Geometry: final body of the model. Coordinates: model frame, mm. Give positions to 0.01 mm unless a question says otherwise; leave off trailing zeros. Order: outer loops, then holes, each group sorted by start corner. A loop starts at its lowest first (then second) coordinate and runs counter-clockwise, first axis right, second up. Notation, with made-up numbers: M 69.25,-34 L 104.25,-34 A18 ccw 104.25,-12 Z; hole C 36.25,5 d10. An arc over 180 degrees is marked long. Use CSV: the item, a comma, the result in double quotes.
```python
from build123d import *

# Parameters (mm, degrees)
SKETCH1_W           = 50.8
SKETCH1_H           = 127
BOSS_EXTRUDE1_DEPTH = 6.35
SKETCH2_R           = 5.08
CUT_EXTRUDE1_DEPTH  = 137.930502446
SKETCH3_W           = 19.05
SKETCH3_H           = 6.35
SKETCH3_R           = 1.524
BOSS_EXTRUDE2_DEPTH = 6.35
BOSS_EXTRUDE3_DEPTH = 6.35
SKETCH5_R           = 1.524
CUT_EXTRUDE2_DEPTH  = 146.219377151


with BuildPart() as part:
    # Sketch1 → Boss-Extrude1 (new body)
    with BuildSketch(Plane.XY):
        with Locations((25.4, 63.5)):
            Rectangle(SKETCH1_W, SKETCH1_H)
    extrude(amount=BOSS_EXTRUDE1_DEPTH)

    # Sketch2 → Cut-Extrude1 (cut, through all)
    with BuildSketch(Plane.XY.offset(6.35)):
        with Locations(Location((6.35, 98.072222222, 0), (0, 0, 180))):
            Circle(SKETCH2_R)
        with Locations(Location((19.05, 98.072222222, 0), (0, 0, 180))):
            Circle(SKETCH2_R)
        with Locations(Location((31.75, 98.072222222, 0), (0, 0, 180))):
            Circle(SKETCH2_R)
        with Locations(Location((44.45, 98.072222222, 0), (0, 0, 180))):
            Circle(SKETCH2_R)
        with Locations(Location((12.7, 86.783333333, 0), (0, 0, 180))):
            Circle(SKETCH2_R)
        with Locations(Location((25.4, 86.783333333, 0), (0, 0, 180))):
            Circle(SKETCH2_R)
        with Locations(Location((38.1, 86.783333333, 0), (0, 0, 180))):
            Circle(SKETCH2_R)
        with Locations(Location((44.45, 75.494444444, 0), (0, 0, 180))):
            Circle(SKETCH2_R)
        with Locations(Location((31.75, 75.494444444, 0), (0, 0, 180))):
            Circle(SKETCH2_R)
        with Locations(Location((19.05, 75.494444444, 0), (0, 0, 180))):
            Circle(SKETCH2_R)
        with Locations(Location((6.35, 75.494444444, 0), (0, 0, 180))):
            Circle(SKETCH2_R)
        with Locations(Location((6.35, 30.338888889, 0), (0, 0, 180))):
            Circle(SKETCH2_R)
        with Locations(Location((19.05, 30.338888889, 0), (0, 0, 180))):
            Circle(SKETCH2_R)
        with Locations(Location((31.75, 30.338888889, 0), (0, 0, 180))):
            Circle(SKETCH2_R)
        with Locations((19.05, 120.65)):
            Circle(SKETCH2_R)
        with Locations((6.35, 120.65)):
            Circle(SKETCH2_R)
        with Locations((31.75, 120.65)):
            Circle(SKETCH2_R)
        with Locations((44.45, 120.65)):
            Circle(SKETCH2_R)
        with Locations((25.4, 109.361111111)):
            Circle(SKETCH2_R)
        with Locations((38.1, 109.361111111)):
            Circle(SKETCH2_R)
        with Locations((12.7, 109.361111111)):
            Circle(SKETCH2_R)
        with Locations(Location((44.45, 30.338888889, 0), (0, 0, 180))):
            Circle(SKETCH2_R)
        with Locations(Location((38.1, 41.627777778, 0), (0, 0, 180))):
            Circle(SKETCH2_R)
        with Locations(Location((25.4, 41.627777778, 0), (0, 0, 180))):
            Circle(SKETCH2_R)
        with Locations(Location((12.7, 41.627777778, 0), (0, 0, 180))):
            Circle(SKETCH2_R)
        with Locations((38.1, 64.205555556)):
            Circle(SKETCH2_R)
        with Locations((25.4, 64.205555556)):
            Circle(SKETCH2_R)
        with Locations((12.7, 64.205555556)):
            Circle(SKETCH2_R)
        with Locations((44.45, 52.916666667)):
            Circle(SKETCH2_R)
        with Locations((31.75, 52.916666667)):
            Circle(SKETCH2_R)
        with Locations((19.05, 52.916666667)):
            Circle(SKETCH2_R)
        with Locations((6.35, 52.916666667)):
            Circle(SKETCH2_R)
        with Locations((12.7, 19.05)):
            Circle(SKETCH2_R)
        with Locations((25.4, 19.05)):
            Circle(SKETCH2_R)
        with Locations((38.1, 19.05)):
            Circle(SKETCH2_R)
        with Locations(Location((6.35, 7.761111111, 0), (0, 0, 180))):
            Circle(SKETCH2_R)
        with Locations(Location((19.05, 7.761111111, 0), (0, 0, 180))):
            Circle(SKETCH2_R)
        with Locations(Location((31.75, 7.761111111, 0), (0, 0, 180))):
            Circle(SKETCH2_R)
        with Locations(Location((44.45, 7.761111111, 0), (0, 0, 180))):
            Circle(SKETCH2_R)
    extrude(amount=-CUT_EXTRUDE1_DEPTH, mode=Mode.SUBTRACT)



with BuildPart() as body_2:
    # Sketch3 → Boss-Extrude2 (new body)
    with BuildSketch(Plane.XY.offset(6.35)):
        with Locations((25.4, -3.175)):
            Rectangle(SKETCH3_W, SKETCH3_H)
        with Locations((25.4, -3.175)):
            Circle(SKETCH3_R, mode=Mode.SUBTRACT)
    extrude(amount=-BOSS_EXTRUDE2_DEPTH)


with BuildPart() as part_1:
    add(part.part)

    add(body_2.part)  # Boss-Extrude3 merges body 2
    # Sketch4 → Boss-Extrude3 (add)
    with BuildSketch(Plane.XY.offset(6.35)):
        Polygon((50.8, 127), (50.8, 0), (57.15, 0), (57.15, 130.175), (57.15, 133.35), (-6.35, 133.35), (-6.35, 127), (-6.35, 0), (0, 0), (0, 127), align=None)
    extrude(amount=-BOSS_EXTRUDE3_DEPTH)

    # Sketch5 → Cut-Extrude2 (cut, through all)
    with BuildSketch(Plane.XY.offset(6.35)):
        with Locations((25.4, 130.175)):
            Circle(SKETCH5_R)
    extrude(amount=-CUT_EXTRUDE2_DEPTH, mode=Mode.SUBTRACT)


solid = part_1.part
```
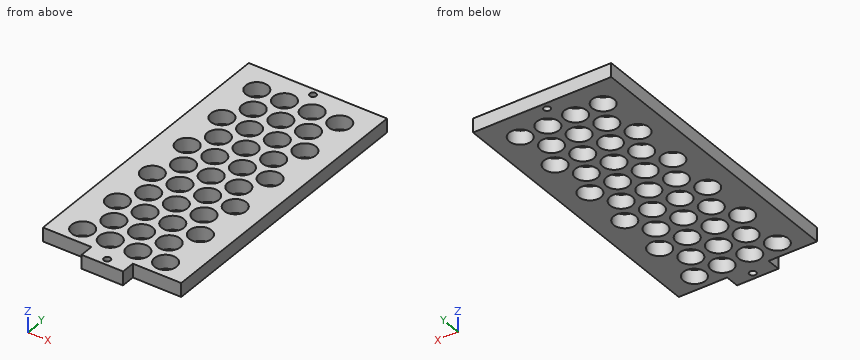
1. Section B-B, the plane x = 25.4. Give the number of separate pieces and of enclosed holes in the cut face, plus the area to 3 significant figures.
Answer:
separate pieces,"8"
enclosed holes,"0"
area,"526 mm2"
2. Section C-C, the plane y = 19.05. Return the cut outline in (x, z), plus the area to 3 significant figures.
Answer:
outline,"M -6.35,0 L 7.62,0 L 7.62,6.35 L -6.35,6.35 Z; M 17.78,0 L 20.32,0 L 20.32,6.35 L 17.78,6.35 Z; M 30.48,0 L 33.02,0 L 33.02,6.35 L 30.48,6.35 Z; M 43.18,0 L 57.15,0 L 57.15,6.35 L 43.18,6.35 Z"
area,"210 mm2"
3. Section A-A, the plane x = 38.1. Return the cut outline in (y, z).
Answer:
outline,"M 0,0 L 13.97,0 L 13.97,6.35 L 0,6.35 Z; M 24.13,0 L 36.55,0 L 36.55,6.35 L 24.13,6.35 Z; M 46.71,0 L 59.13,0 L 59.13,6.35 L 46.71,6.35 Z; M 69.29,0 L 81.7,0 L 81.7,6.35 L 69.29,6.35 Z; M 91.86,0 L 104.28,0 L 104.28,6.35 L 91.86,6.35 Z; M 114.44,0 L 133.35,0 L 133.35,6.35 L 114.44,6.35 Z"
4. Pin query (flat end, axial travel): pin 1 Ø6 at (x, y) = (31.75, 30.34) entering from +Z; pin 2 Ø3.5 at (x, y) = (25.4, 130.175) entering from -Z; pin 3 Ø3 at (x, z) = (13.5, 3) entering from -Y. Return the tip coordinate at first contact, or that it passes through.
Answer:
pin 1,"through"
pin 2,"z = 0"
pin 3,"y = 0"
5. Line query: line 1 (X direction, y = 29, z = 0.75); line 2 (X direction, y = 82.5, z = 4.5); line 3 (X direction, y = 53, z = 2). Output: solid intervals per line, ascending.
Answer:
line 1,"-6.35 to 1.45, 11.25 to 14.15, 23.95 to 26.85, 36.65 to 39.55, 49.35 to 57.15"
line 2,"-6.35 to 9.97, 15.43 to 22.67, 28.13 to 35.37, 40.83 to 57.15"
line 3,"-6.35 to 1.27, 11.43 to 13.97, 24.13 to 26.67, 36.83 to 39.37, 49.53 to 57.15"
6. Section D-D, the plane x = 6.35. Return the cut outline in (y, z), plus the area to 3 significant figures.
Answer:
outline,"M 0,0 L 2.68,0 L 2.68,6.35 L 0,6.35 Z; M 12.84,0 L 25.26,0 L 25.26,6.35 L 12.84,6.35 Z; M 35.42,0 L 47.84,0 L 47.84,6.35 L 35.42,6.35 Z; M 58,0 L 70.41,0 L 70.41,6.35 L 58,6.35 Z; M 80.57,0 L 92.99,0 L 92.99,6.35 L 80.57,6.35 Z; M 103.15,0 L 115.57,0 L 115.57,6.35 L 103.15,6.35 Z; M 125.73,0 L 133.35,0 L 133.35,6.35 L 125.73,6.35 Z"
area,"460 mm2"
